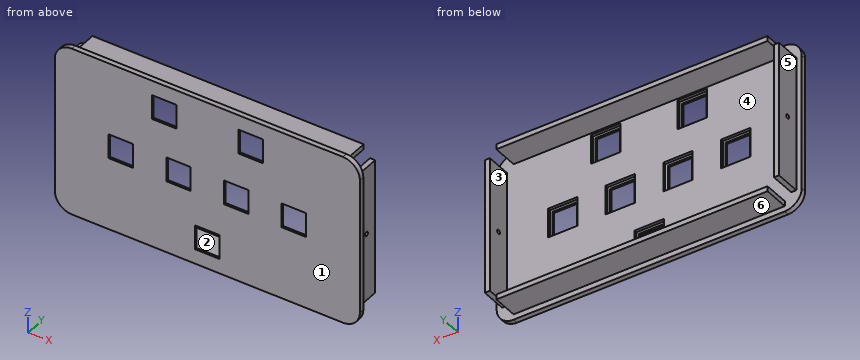
Autodesk Fusion 360 part; units mm, degrees
sketch "Top" plane through (0, 0, 0) normal (0, 1, 0) x (1, 0, 0)
  line L0 (-80, 50) -> (80, 50)
  line L1 (90, 40) -> (90, -40)
  line L2 (80, -50) -> (-80, -50)
  line L3 (-90, -40) -> (-90, 40)
  line L4 (-90, 50) -> (90, -50) construction
  line L5 (90, 50) -> (-90, -50) construction
  arc A0 (-80, 50) -> (-90, 40) centre (-80, 40) ccw
  arc A1 (90, 40) -> (80, 50) centre (80, 40) ccw
  arc A2 (80, -50) -> (90, -40) centre (80, -40) ccw
  arc A3 (-90, -40) -> (-80, -50) centre (-80, -40) ccw
  dimension "d310" = 180
  dimension "d311" = 100
  dimension "d312" = 10
extrude "Extrude37" add sketch "Top" along normal blind 3
sketch "Tabs" plane through (0, 3, 0) normal (0, 1, 0) x (-1, 0, 0)
  arc A0 (80, -50) -> (90, -40) centre (80, -40) ccw
  line L0 (90, -40) -> (90, 40)
  arc A1 (90, 40) -> (80, 50) centre (80, 40) ccw
  line L1 (80, 50) -> (-80, 50)
  arc A2 (-80, 50) -> (-90, 40) centre (-80, 40) ccw
  line L2 (-90, 40) -> (-90, -40)
  arc A3 (-90, -40) -> (-80, -50) centre (-80, -40) ccw
  line L3 (-80, -50) -> (80, -50)
  line L4 (86.8, -40) -> (83.8, -40)
  line L5 (83.8, -40) -> (83.8, 40)
  line L6 (83.8, 40) -> (86.8, 40)
  line L7 (86.8, 40) -> (86.8, -40)
  line L8 (86.8, -40) -> (83.8, 40) construction
  line L9 (83.8, -40) -> (86.8, 40) construction
  line L10 (80, -46.8) -> (-80, -46.8)
  line L11 (-80, -46.8) -> (-80, -43.8)
  line L12 (-80, -43.8) -> (80, -43.8)
  line L13 (80, -43.8) -> (80, -46.8)
  line L14 (80, -46.8) -> (-80, -43.8) construction
  line L15 (-80, -46.8) -> (80, -43.8) construction
  line L16 (80, 43.8) -> (-80, 43.8)
  line L17 (-80, 43.8) -> (-80, 46.8)
  line L18 (-80, 46.8) -> (80, 46.8)
  line L19 (80, 46.8) -> (80, 43.8)
  line L20 (80, 43.8) -> (-80, 46.8) construction
  line L21 (-80, 43.8) -> (80, 46.8) construction
  line L22 (-83.8, -40) -> (-86.8, -40)
  line L23 (-86.8, -40) -> (-86.8, 40)
  line L24 (-86.8, 40) -> (-83.8, 40)
  line L25 (-83.8, 40) -> (-83.8, -40)
  line L26 (-83.8, -40) -> (-86.8, 40) construction
  line L27 (-86.8, -40) -> (-83.8, 40) construction
  point P0 (85.3, 0)
  point P1 (0, -45.3)
  point P2 (0, 45.3)
  point P3 (-85.3, 0)
  dimension "d315" = 3
  dimension "d316" = 10
  dimension "d317" = 10
  dimension "d318" = 3.2
  dimension "d319" = 3
  dimension "d320" = 10
  dimension "d321" = 10
  dimension "d322" = 3.2
  dimension "d324" = 3
  dimension "d325" = 10
  dimension "d326" = 10
  dimension "d327" = 3
  dimension "d329" = 10
  dimension "d330" = 10
  dimension "d333" = 3.2
  dimension "d334" = 3.2
extrude "Extrude38" add sketch "Tabs" along normal blind 15 contours L4 L5 L6 L7 | L10 L11 L12 L13 | L16 L17 L18 L19 | L22 L23 L24 L25
sketch "Switches" plane through (0, 3, 0) normal (0, 1, 0) x (-1, 0, 0)
  line L0 (86.8, 40) -> (86.8, -40)
  line L1 (86.8, -40) -> (83.8, -40)
  line L2 (83.8, -40) -> (83.8, 40)
  line L3 (83.8, 40) -> (86.8, 40)
  line L4 (80, -43.8) -> (80, -46.8)
  line L5 (80, -46.8) -> (-80, -46.8)
  line L6 (-80, -46.8) -> (-80, -43.8)
  line L7 (-80, -43.8) -> (80, -43.8)
  line L8 (80, 46.8) -> (80, 43.8)
  line L9 (80, 43.8) -> (-80, 43.8)
  line L10 (-80, 43.8) -> (-80, 46.8)
  line L11 (-80, 46.8) -> (80, 46.8)
  line L12 (-83.8, 40) -> (-83.8, -40)
  line L13 (-83.8, -40) -> (-86.8, -40)
  line L14 (-86.8, -40) -> (-86.8, 40)
  line L15 (-86.8, 40) -> (-83.8, 40)
  arc A0 (80, -50) -> (90, -40) centre (80, -40) ccw
  line L16 (90, -40) -> (90, 40)
  arc A1 (90, 40) -> (80, 50) centre (80, 40) ccw
  line L17 (80, 50) -> (-80, 50)
  arc A2 (-80, 50) -> (-90, 40) centre (-80, 40) ccw
  line L18 (-90, 40) -> (-90, -40)
  arc A3 (-90, -40) -> (-80, -50) centre (-80, -40) ccw
  line L19 (-80, -50) -> (80, -50)
  line L20 (-59.7, 8.7) -> (-42.3, 8.7)
  line L21 (-42.3, 8.7) -> (-42.3, -8.7)
  line L22 (-58.2, -7.2) -> (-58.2, 7.2)
  line L23 (-42.3, -8.7) -> (-59.7, -8.7)
  line L24 (-43.8, 7.2) -> (-43.8, -7.2)
  line L25 (-58.2, 7.2) -> (-43.8, 7.2)
  line L26 (-43.8, -7.2) -> (-58.2, 7.2) construction
  line L27 (-59.7, -8.7) -> (-59.7, 8.7)
  line L28 (-59.7, -8.7) -> (-42.3, 8.7) construction
  line L29 (-58.2, -7.2) -> (-43.8, 7.2) construction
  line L30 (-42.3, -8.7) -> (-59.7, 8.7) construction
  line L31 (-43.8, -7.2) -> (-58.2, -7.2)
  line L32 (24.2, 7.2) -> (24.2, -7.2)
  line L33 (8.3, -8.7) -> (8.3, 8.7)
  line L34 (25.7, -8.7) -> (8.3, 8.7) construction
  line L35 (9.8, 7.2) -> (24.2, 7.2)
  line L36 (24.2, -7.2) -> (9.8, 7.2) construction
  line L37 (8.3, -8.7) -> (25.7, 8.7) construction
  line L38 (9.8, -7.2) -> (24.2, 7.2) construction
  line L39 (24.2, -7.2) -> (9.8, -7.2)
  line L40 (25.7, 8.7) -> (25.7, -8.7)
  line L41 (9.8, -7.2) -> (9.8, 7.2)
  line L42 (25.7, -8.7) -> (8.3, -8.7)
  line L43 (8.3, 8.7) -> (25.7, 8.7)
  line L44 (-18.3, 26.9) -> (-32.7, 41.3) construction
  line L45 (-32.7, 41.3) -> (-18.3, 41.3)
  line L46 (-16.8, 25.4) -> (-34.2, 25.4)
  line L47 (-34.2, 42.8) -> (-16.8, 42.8)
  line L48 (-32.7, 26.9) -> (-32.7, 41.3)
  line L49 (-16.8, 42.8) -> (-16.8, 25.4)
  line L50 (-34.2, 25.4) -> (-34.2, 42.8)
  line L51 (-16.8, 25.4) -> (-34.2, 42.8) construction
  line L52 (-18.3, 26.9) -> (-32.7, 26.9)
  line L53 (-32.7, 26.9) -> (-18.3, 41.3) construction
  line L54 (-34.2, 25.4) -> (-16.8, 42.8) construction
  line L55 (-18.3, 41.3) -> (-18.3, 26.9)
  line L56 (16.8, 25.4) -> (34.2, 42.8) construction
  line L57 (18.3, 41.3) -> (32.7, 41.3)
  line L58 (34.2, 42.8) -> (34.2, 25.4)
  line L59 (18.3, 26.9) -> (32.7, 41.3) construction
  line L60 (32.7, 26.9) -> (18.3, 26.9)
  line L61 (16.8, 25.4) -> (16.8, 42.8)
  line L62 (32.7, 41.3) -> (32.7, 26.9)
  line L63 (16.8, 42.8) -> (34.2, 42.8)
  line L64 (34.2, 25.4) -> (16.8, 42.8) construction
  line L65 (34.2, 25.4) -> (16.8, 25.4)
  line L66 (18.3, 26.9) -> (18.3, 41.3)
  line L67 (32.7, 26.9) -> (18.3, 41.3) construction
  line L68 (-8.7, -42.8) -> (-8.7, -25.4)
  line L69 (-7.2, -41.3) -> (-7.2, -26.9)
  line L70 (7.2, -26.9) -> (7.2, -41.3)
  line L71 (-7.2, -41.3) -> (7.2, -26.9) construction
  line L72 (8.7, -25.4) -> (8.7, -42.8)
  line L73 (8.7, -42.8) -> (-8.7, -42.8)
  line L74 (7.2, -41.3) -> (-7.2, -26.9) construction
  line L75 (8.7, -42.8) -> (-8.7, -25.4) construction
  line L76 (-8.7, -42.8) -> (8.7, -25.4) construction
  line L77 (-8.7, -25.4) -> (8.7, -25.4)
  line L78 (7.2, -41.3) -> (-7.2, -41.3)
  line L79 (-7.2, -26.9) -> (7.2, -26.9)
  line L80 (42.3, -8.7) -> (42.3, 8.7)
  line L81 (43.8, 7.2) -> (58.2, 7.2)
  line L82 (42.3, 8.7) -> (59.7, 8.7)
  line L83 (59.7, -8.7) -> (42.3, -8.7)
  line L84 (58.2, -7.2) -> (43.8, -7.2)
  line L85 (58.2, 7.2) -> (58.2, -7.2)
  line L86 (42.3, -8.7) -> (59.7, 8.7) construction
  line L87 (59.7, -8.7) -> (42.3, 8.7) construction
  line L88 (43.8, -7.2) -> (43.8, 7.2)
  line L89 (43.8, -7.2) -> (58.2, 7.2) construction
  line L90 (58.2, -7.2) -> (43.8, 7.2) construction
  line L91 (59.7, 8.7) -> (59.7, -8.7)
  line L92 (-25.7, 8.7) -> (-8.3, 8.7)
  line L93 (-25.7, -8.7) -> (-8.3, 8.7) construction
  line L94 (-25.7, -8.7) -> (-25.7, 8.7)
  line L95 (-9.8, 7.2) -> (-9.8, -7.2)
  line L96 (-9.8, -7.2) -> (-24.2, -7.2)
  line L97 (-8.3, -8.7) -> (-25.7, 8.7) construction
  line L98 (-24.2, -7.2) -> (-9.8, 7.2) construction
  line L99 (-8.3, -8.7) -> (-25.7, -8.7)
  line L100 (-24.2, -7.2) -> (-24.2, 7.2)
  line L101 (-9.8, -7.2) -> (-24.2, 7.2) construction
  line L102 (-8.3, 8.7) -> (-8.3, -8.7)
  line L103 (-24.2, 7.2) -> (-9.8, 7.2)
  point P0 (-51, 0)
  point P1 (17, 0)
  point P2 (-25.5, 34.1)
  point P3 (25.5, 34.1)
  point P4 (0, -34.1)
  point P5 (51, 0)
  point P6 (-17, 0)
  dimension "d345" = 14.4
  dimension "d346" = 14.4
  dimension "d347" = 1.5
  dimension "d348" = 1.5
  dimension "d349" = 1.5
  dimension "d350" = 1.5
  dimension "d363" = 14.4
  dimension "d364" = 14.4
  dimension "d365" = 1.5
  dimension "d366" = 1.5
  dimension "d367" = 1.5
  dimension "d368" = 1.5
  dimension "d369" = 14.4
  dimension "d370" = 14.4
  dimension "d371" = 1.5
  dimension "d372" = 1.5
  dimension "d373" = 1.5
  dimension "d374" = 1.5
  dimension "d375" = 14.4
  dimension "d376" = 14.4
  dimension "d377" = 1.5
  dimension "d378" = 1.5
  dimension "d379" = 1.5
  dimension "d380" = 1.5
  dimension "d381" = 14.4
  dimension "d382" = 14.4
  dimension "d383" = 1.5
  dimension "d384" = 1.5
  dimension "d385" = 1.5
  dimension "d386" = 1.5
  dimension "d387" = 14.4
  dimension "d388" = 14.4
  dimension "d389" = 1.5
  dimension "d390" = 1.5
  dimension "d391" = 1.5
  dimension "d392" = 1.5
  dimension "d393" = 14.4
  dimension "d394" = 14.4
  dimension "d395" = 1.5
  dimension "d396" = 1.5
  dimension "d397" = 1.5
  dimension "d398" = 1.5
  dimension "d399" = 1
  dimension "d400" = 1
  dimension "d401" = 1
  dimension "d404" = 51
  dimension "d405" = 25.5
  dimension "d406" = 34
  dimension "d407" = 34
  dimension "d408" = 34
  dimension "d409" = 17
extrude "Extrude40" cut sketch "Switches" against normal blind 1.7 contours L20 L21 L23 L27 | L33 L40 L42 L43 | L46 L47 L49 L50 | L58 L61 L63 L65 | L68 L72 L73 L77 | L80 L82 L83 L91 | L92 L94 L99 L102
extrude "Extrude41" cut sketch "Switches" along normal blind 3 from surface at -3 contours L22 L24 L25 L31 | L32 L35 L39 L41 | L45 L48 L52 L55 | L57 L60 L62 L66 | L69 L70 L78 L79 | L81 L84 L85 L88 | L95 L96 L100 L103
sketch "Tab Holes" plane through (0, 0, 0) normal (1, 0, 0) x (0, 0, -1)
  circle A0 centre (0, 10.5) radius 1.25
  line L0 (-40, 3) -> (40, 3)
  dimension "d418" = 2.5
  dimension "d419" = 7.5
extrude "Extrude42" cut sketch "Tab Holes" along normal through all and the other way through all
equation "d405 = ( 51 / 2 ) * 1 mm"
equation "d409 = ( 34 / 2 ) * 1 mm"
equation "d413 = -( 3 mm - 1.3 mm )"
equation "d419 = ( 15 / 2 ) * 1 mm"
Build history of the part. All positions in model axes, mm. Face numbers are marked on the shaded views. A direction names the side the tool comes from. Round coordinates to 2 decimals unless told otherwise and drop trailing zeros. Loops run counter-clockwise (first coordinate to the right, second up) from the corner with the lowest first, then second, coordinate; pieces in that order, holes last.
Item 1: Saw through at A-A (x = 47). List the corners of the cut face in (y, z).
Item 2: Saw through at D-D (x = -22.5). List the corners of the cut face in (y, z).
Item 3: Drill centre lines: line 1 along X through (y, z) = (2, 6); line 2 along X through (y, z) = (15.25, 15); line 3 along Y through (x, z) = (85, 0). Where is each one in solid material? Low to high.
Item 4: Saw through at B-B (z = 35.5). List the corners of the cut face in (x, y).
Item 5: Which spindle directions (+Z, -Z, +X, -X, +Y, -Y) get a long thin tool onto all of the face, cutting with end or side? Do the marked faces 1, 2 and 3. Say none if no direction does.
Item 6: Pin check, flat tips, straight feed: P1, Ø1, axis at x = -21, z = -25, coming from the +Y side; P2, Ø7.5, axis at y = 13, z = 13.5, coming from the +X side; P3, Ø10, axis at x = -14, z = -1.5, coming from the +Y side; P4, Ø2, axis at x = -11, z = -4, coming from the -Y side. Stop position of each tip, or through.
Item 7: Two-plate mould, pull along X, no slides. Class the marked faces 4, 5 and 6: released by +X, released by -X, zero draft, split by the parting line, or undercut.
Item 8: Saw through at C-C (y = 5.25). List the corners of the cut face in (x, z), then the cut area to 3 significant figures.
Worked answers:
1. outline: (0, -50) - (3, -50) - (3, -46.8) - (18, -46.8) - (18, -43.8) - (3, -43.8) - (3, -8.7) - (1.3, -8.7) - (1.3, -7.2) - (0, -7.2) - close; (0, 7.2) - (1.3, 7.2) - (1.3, 8.7) - (3, 8.7) - (3, 43.8) - (18, 43.8) - (18, 46.8) - (3, 46.8) - (3, 50) - (0, 50) - close
2. outline: (0, -50) - (3, -50) - (3, -46.8) - (18, -46.8) - (18, -43.8) - (3, -43.8) - (3, -8.7) - (1.3, -8.7) - (1.3, -7.2) - (0, -7.2) - close; (0, 7.2) - (1.3, 7.2) - (1.3, 8.7) - (3, 8.7) - (3, 25.4) - (1.3, 25.4) - (1.3, 26.9) - (0, 26.9) - close; (0, 41.3) - (1.3, 41.3) - (1.3, 42.8) - (3, 42.8) - (3, 43.8) - (18, 43.8) - (18, 46.8) - (3, 46.8) - (3, 50) - (0, 50) - close
3. line 1: x = -90 to -59.7, -42.3 to -25.7, -8.3 to 8.3, 25.7 to 42.3, 59.7 to 90
3. line 2: x = -86.8 to -83.8, 83.8 to 86.8
3. line 3: y = 0 to 9.25, 11.75 to 18
4. outline: (-90, 0) - (-32.7, 0) - (-32.7, 1.3) - (-34.2, 1.3) - (-34.2, 3) - (-83.8, 3) - (-83.8, 18) - (-86.8, 18) - (-86.8, 3) - (-90, 3) - close; (-18.3, 0) - (18.3, 0) - (18.3, 1.3) - (16.8, 1.3) - (16.8, 3) - (-16.8, 3) - (-16.8, 1.3) - (-18.3, 1.3) - close; (32.7, 0) - (90, 0) - (90, 3) - (86.8, 3) - (86.8, 18) - (83.8, 18) - (83.8, 3) - (34.2, 3) - (34.2, 1.3) - (32.7, 1.3) - close
5. face 1: +Z, -Z, +X, -X, -Y
5. face 2: +X, -X, +Y
5. face 3: +Z, -Z, +Y
6. P1: stops at y = 3
6. P2: stops at x = 86.8
6. P3: stops at y = 1.3
6. P4: passes through
7. face 4: undercut
7. face 5: released by -X
7. face 6: zero draft
8. outline: (-86.8, -40) - (-83.8, -40) - (-83.8, 40) - (-86.8, 40) - close; (-80, -46.8) - (80, -46.8) - (80, -43.8) - (-80, -43.8) - close; (-80, 43.8) - (80, 43.8) - (80, 46.8) - (-80, 46.8) - close; (83.8, -40) - (86.8, -40) - (86.8, 40) - (83.8, 40) - close
8. area: 1,440 mm2
